from build123d import *

# Parameters (mm, degrees)
F0_W      = 19.05
F0_H      = 19.05
F1_DEPTH  = 19.05
F1_FACE_W = 19.05
F1_FACE_H = 19.05
F2_DEPTH  = 38.1
F3_W      = 19.05
F3_H      = 19.05
F4_DEPTH  = 38.1


with BuildPart() as f1:
    # F0 (on Top) → F1 (new body)
    with BuildSketch(Plane.XY):
        with Locations((9.525, -9.525)):
            Rectangle(F0_W, F0_H)
    extrude(amount=F1_DEPTH)

    # F1_face (on face) → F2 (join)
    with BuildSketch(Plane(origin=(9.525, -19.05, 9.525), x_dir=(1, 0, 0), z_dir=(0, -1, 0))):
        Rectangle(F1_FACE_W, F1_FACE_H)
    extrude(amount=F2_DEPTH)

    # F3 (on face) → F4 (join)
    with BuildSketch(Plane.YZ.offset(19.05)):
        with Locations((-9.525, 9.525)):
            Rectangle(F3_W, F3_H)
    extrude(amount=F4_DEPTH)


solid = f1.part
Work out the finished part from the listing and answer in its coordinate system (mm). A direction names the side the tool comes from. Round coordinates to 2 decimals unless told otherwise and drop trailing zeros. Order: outer loops, then holes, each group sorted by start corner. A loop starts at its lowest first (then second) coordinate and runs counter-clockwise, first axis right, second up. Notation, with made-up numbers: M 54,51 L 77,51 A20 ccw 77,78 Z; hole C 81.25,-20 d2. An arc over 180 degrees is marked long. One line per item, written item: value.
Q1. Flat-ended cylindrical pins translate along their axes: pin 1 (1.5 mm diameter, centred on x = 47.5, z = 6.5, fed in from -Y); pin 2 (1 mm diameter, centred on y = -49.5, z = 8.5, fed in from +X). Find the tip coordinate at first contact, or state that the pin passes through.
Derived:
pin 1: y = -19.05
pin 2: x = 19.05
Q2. Straight lines are drawn through the part: line 1 (X direction, y = -46, z = 15); line 2 (Y direction, x = 38, z = 1.5). For each, find the intervals that lie inside material, in ascending order.
Derived:
line 1: 0 to 19.05
line 2: -19.05 to 0
Q3. Find section C-C on y = -50. Write down the section's boundary in (x, z), then the cut area to 3 significant figures.
Derived:
outline: M 0,0 L 19.05,0 L 19.05,19.05 L 0,19.05 Z
area: 363 mm²
Q4. Find section A-A on z = 10.25. Write down the section's boundary in (x, y).
Derived:
outline: M 0,-57.15 L 19.05,-57.15 L 19.05,-19.05 L 57.15,-19.05 L 57.15,0 L 0,0 Z
Q5. For faces 1 (the face through (38, -19.05, 9)), 2 (the face through (57.15, -10, 10)), determine the directions among +Z, -Z, +X, -X, +Y, -Y from which every point of the face is accessible in a straight line to the end or side of a thin tool.
Derived:
face 1: +Z, -Z, +X, -Y
face 2: +Z, -Z, +X, +Y, -Y
Q6. Find section B-B on x = 29. Write down the section's boundary in (y, z).
Derived:
outline: M -19.05,0 L 0,0 L 0,19.05 L -19.05,19.05 Z
